Input: dimensioned drawing with shaded views. Units: mm. Origin: part minimum x, y, z. A direction names the side the tool comes from. Round coordinates to 2 decimals unless told otherwise and drop trailing zeros. Loops run counter-clockwise (first coordinate to the right, second up) from the corner with the lowest first, then second, coordinate; pieces in that order, holes last. Notation, with made-up numbers: (47, -25.75) - (63, -25.75) arc R16 ccw to (63, -19.75) - close; hole circle Ø5 at (-16.75, -40). An arc over 180 degrees is marked (long way). One line per question, with ' | ' between items.
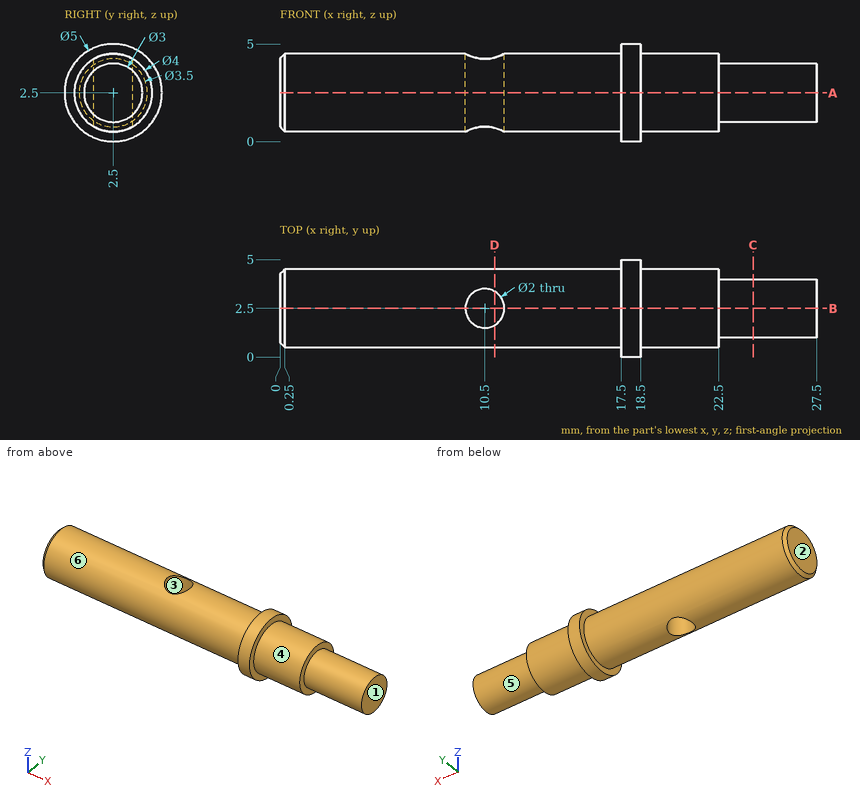
1. Section query B-B, the plane y = 2.5. Return loops of the section in (x, z).
Worked out:
outline: (0, 0.75) - (0.25, 0.5) - (9.5, 0.5) - (9.5, 4.5) - (0.25, 4.5) - (0, 4.25) - close; (11.5, 0.5) - (17.5, 0.5) - (17.5, 0) - (18.5, 0) - (18.5, 0.5) - (22.5, 0.5) - (22.5, 1) - (27.5, 1) - (27.5, 4) - (22.5, 4) - (22.5, 4.5) - (18.5, 4.5) - (18.5, 5) - (17.5, 5) - (17.5, 4.5) - (11.5, 4.5) - close
2. Contact query for flat-ended pins moving along their axis: P1, Ø1.5, axis at x = 16, z = 1, coming from the +Y side; P2, Ø2.5, axis at x = 10.5, y = 2.5, coming from the +Z side; P3, Ø2, axis at y = 3.5, z = 1.5, coming from the -X side; P4, Ø1, axis at x = 13.5, y = 4.5, coming from the +Z side. Output: stop coordinate, or through.
Worked out:
P1: stops at y = 4.35 | P2: stops at z = 4.5 | P3: stops at x = 0 | P4: stops at z = 3.82
3. Section query C-C, the plane x = 24.25. Return loops of the section in (y, z), plus the area to 3 significant figures.
Worked out:
outline: circle Ø3 at (2.5, 2.5) | area: 7.07 mm2
4. Access query for the marked faces 5 and 6. Directions: +Z, -Z, +X, -X, +Y, -Y. A direction counts if a zero-diameter tool reaches every point of the face in a straight line with its end or side. Return the directions, or none.
Worked out:
face 5: +X | face 6: -X
5. Section query A-A, the plane z = 2.5. Return loops of the section in (x, y).
Worked out:
outline: (0, 0.75) - (0.25, 0.5) - (17.5, 0.5) - (17.5, 0) - (18.5, 0) - (18.5, 0.5) - (22.5, 0.5) - (22.5, 1) - (27.5, 1) - (27.5, 4) - (22.5, 4) - (22.5, 4.5) - (18.5, 4.5) - (18.5, 5) - (17.5, 5) - (17.5, 4.5) - (0.25, 4.5) - (0, 4.25) - close; hole circle Ø2 at (10.5, 2.5)
6. Section query D-D, the plane x = 11. Return loops of the section in (y, z), plus the area to 3 significant figures.
Worked out:
outline: (1.63, 0.7) - (1.63, 4.3) arc R2 ccw to start; (3.37, 0.7) arc R2 ccw to (3.37, 4.3) - close | area: 5.86 mm2
7. Mould query, pull axis X, two halves, no side actions, for the marked faces 1, 2, 3 and 4. Classes: released by +X, released by -X, zero draft, split by the parting line, or undercut.
Worked out:
face 1: released by +X | face 2: released by -X | face 3: undercut | face 4: zero draft
8. Material intervals for probe 1 along X at (y, z) = (2.5, 3.5); probe 2 along Y at (x, z) = (6.25, 2.55); probe 3 along Y at (x, z) = (10.5, 1.9), sorted ascending.
Worked out:
probe 1: x = 0 to 9.5, 11.5 to 27.5 | probe 2: y = 0.5 to 4.5 | probe 3: y = 0.59 to 1.5, 3.5 to 4.41
